Job drawing, mm, ordinate dimensions from the low corner. One solid piece. Coordinates: 2 decimals unless noted, no trailing zeros. Order: outer loops, then holes, each group sorted by start corner. A loop starts at its lowest first (then second) coordinate and runs counter-clockwise, first axis right, second up. Notation, with made-up numbers: (53.25, 16) - (70.25, 16) arc R32 cw to (70.25, 51) - close; hole circle Ø4 at (-25.75, -25.75). An arc over 180 degrees is marked (long way). Return JSON: item names as keys, results as strings.
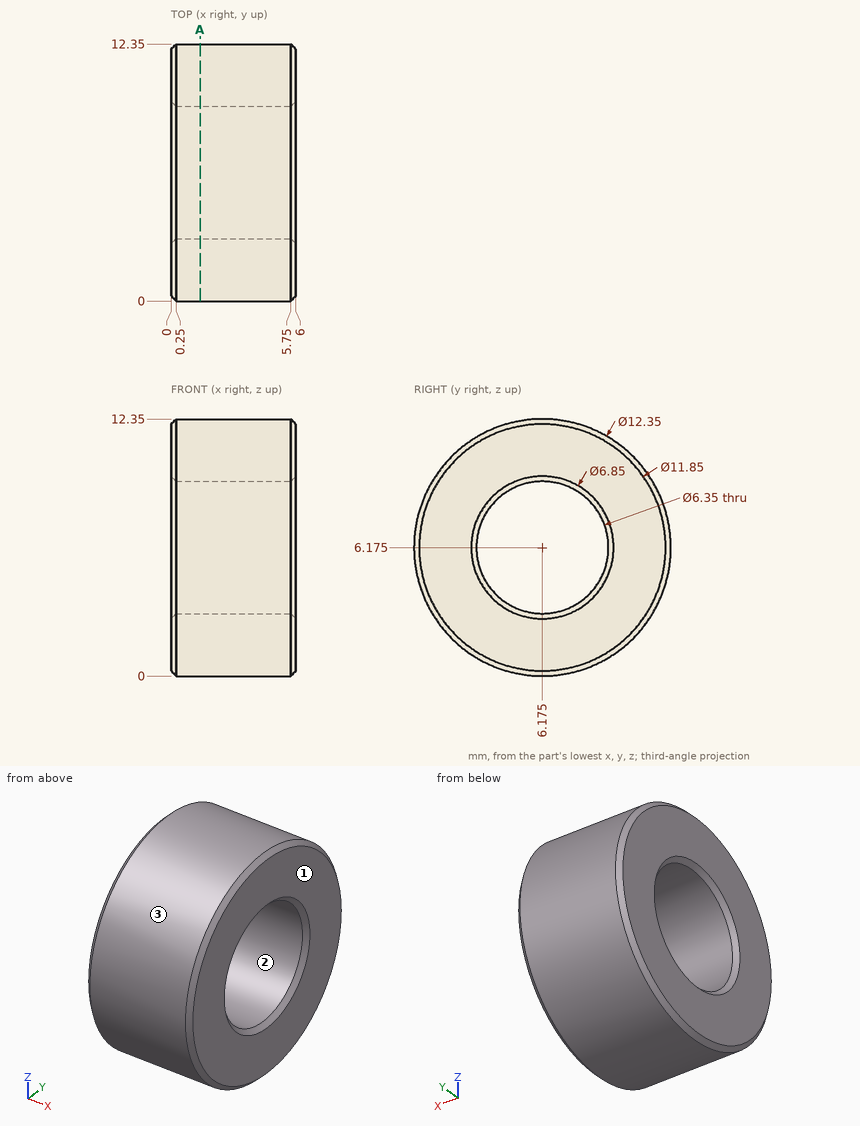
1. Mould opens along Y. For the marked faces 1, 2 and 3 say: pulls with the +Y half, pulls with the -Y half, needs draft (parallel to the pull), parting line crosses it, or undercut.
Check values:
{"face 1": "needs draft", "face 2": "undercut", "face 3": "parting line crosses it"}
2. Drop flat-ended pins along their axis: pin 1 (3 mm diameter, centred on x = 3.5, y = 10, fed in from -Z); pin 2 (1 mm diameter, centred on x = 1, y = 10.5, fed in from -Z). Give the stop position or say it passes through.
Check values:
{"pin 1": "z = 0.45", "pin 2": "z = 1.33"}
3. Cut at A-A on x = 1.4. Give the cut face in (y, z) (3 decimals).
Check values:
{"outline": "circle Ø12.35 at (6.175, 6.175); hole circle Ø6.35 at (6.175, 6.175)"}
4. Probe L1, parallel to Z at x = 3.85, y = 3.75; L2, parallel to Y at x = 4.1, z = 6.25; L3, parallel to Y at x = 0.65, z = 7. List the from-to ranges inside material, lowest first.
Check values:
{"L1": "0.5 to 4.13, 8.22 to 11.85", "L2": "0 to 3, 9.35 to 12.35", "L3": "0.06 to 3.11, 9.24 to 12.29"}
